Design review of the part built by this model. Coordinates are the model's own, in mm. A direction names the side the tool comes from. Round coordinates to 2 decimals unless told otherwise and drop trailing zeros. Write each loop counter-clockwise with the first axis right and the second up, starting at its lowest first coordinate (ties: lowest second). Pieces come first, ordered by that corner, then holes. Notation, with made-up numbers: (78.5, 51) - (98.5, 51) arc R17 cw to (98.5, 58) - close; hole circle Ø3 at (63, -26). An arc over 180 degrees is marked (long way). Use one line per item in the form item = value.
Autodesk Inventor part; units mm, degrees
ref_plane "h1_XY" through (-121.4374, 0, 0) normal (0, 1, 0) x (1, 0, 0)
ref_plane "h1_YZ" through (-121.4374, 0, 0) normal (1, 0, 0) x (0, 0, -1)
ref_plane "h1_ZX" through (-121.4374, 0, 0) normal (0, 0, -1) x (0, 1, 0)
sketch "Sketch_3" plane through (0, 0, 0) normal (0, 0, 1) x (1, 0, 0)
  line L0 (0, 0) -> (-121.4374, 0)
  line L1 (-121.4374, 0) -> (-121.4374, 1.9406)
  line L2 (-121.4374, 1.9406) -> (-120.965, 2.413)
  line L3 (-120.965, 2.413) -> (0, 2.413)
  line L4 (0, 2.413) -> (0, 0)
  line L5 (0, 0) -> (-121.4374, 0)
revolve "Revolution1" add sketch "Sketch_3" angle 360 about axis through (0, 0, 0) along (1, 0, 0)
thread "Thread1"
sketch "Sketch_17" plane through (0, 0, 0) normal (0, 0, 1) x (1, 0, 0)
  line L0 (121.4374, 0) -> (-121.4374, 0)
  line L1 (-108.9914, 2.413) -> (-108.9914, 2.159)
  line L2 (-108.9914, 2.159) -> (-108.7374, 2.159)
  line L3 (-108.7374, 2.159) -> (-108.7374, 2.413)
  line L4 (-108.7374, 2.413) -> (-108.9914, 2.413)
revolve "Revolution2" cut sketch "Sketch_17" angle 360 about axis through (121.4374, 0, 0) along (1, 0, 0)
sketch "Sketch_12" plane through (0, 0, 0) normal (0, 0, 1) x (1, 0, 0)
  line L0 (1.524, 0) -> (-15.875, 0)
  line L1 (-15.875, 0) -> (-15.875, 7.2771)
  line L2 (-15.875, 7.2771) -> (1.524, 7.2771)
  line L3 (1.524, 7.2771) -> (1.524, 0)
  line L4 (1.524, 0) -> (-15.875, 0)
revolve "Revolution3" add sketch "Sketch_12" angle 360 about axis through (1.524, 0, 0) along (1, 0, 0)
ref_plane "h1_XY" through (-121.4374, 0, 0) normal (0, 1, 0) x (1, 0, 0)
ref_plane "h1_YZ" through (-121.4374, 0, 0) normal (1, 0, 0) x (0, 0, -1)
ref_plane "h1_ZX" through (-121.4374, 0, 0) normal (0, 0, -1) x (0, 1, 0)
ref_plane "h2_XY" through (-108.7374, 0, 0) normal (0, 1, 0) x (1, 0, 0)
ref_plane "h2_YZ" through (-108.7374, 0, 0) normal (1, 0, 0) x (0, 0, -1)
ref_plane "h2_ZX" through (-108.7374, 0, 0) normal (0, 0, -1) x (0, 1, 0)
ref_plane "k1_XY" through (-121.4374, 0, -2.413) normal (0, 1, 0) x (1, 0, 0)
ref_plane "k1_YZ" through (-121.4374, 0, -2.413) normal (1, 0, 0) x (0, 0, -1)
ref_plane "k1_ZX" through (-121.4374, 0, -2.413) normal (0, 0, -1) x (0, 1, 0)
ref_plane "k2_XY" through (-121.4374, 0, 2.413) normal (0, 1, 0) x (1, 0, 0)
ref_plane "k2_YZ" through (-121.4374, 0, 2.413) normal (1, 0, 0) x (0, 0, -1)
ref_plane "k2_ZX" through (-121.4374, 0, 2.413) normal (0, 0, -1) x (0, 1, 0)
ref_plane "start_XY" through (-108.7374, 0, 0) normal (0, 1, 0) x (1, 0, 0)
ref_plane "start_YZ" through (-108.7374, 0, 0) normal (1, 0, 0) x (0, 0, -1)
ref_plane "start_ZX" through (-108.7374, 0, 0) normal (0, 0, -1) x (0, 1, 0)
ref_plane "to_prc_XY" through (-108.7374, 0, 0) normal (1, 0, 0) x (0, 0, -1)
ref_plane "to_prc_YZ" through (-108.7374, 0, 0) normal (0, 0, -1) x (0, 1, 0)
ref_plane "to_prc_ZX" through (-108.7374, 0, 0) normal (0, 1, 0) x (1, 0, 0)
ref_plane "to_rod_guide_XY" through (-121.4374, 0, 0) normal (1, 0, 0) x (0, 0, -1)
ref_plane "to_rod_guide_YZ" through (-121.4374, 0, 0) normal (0, 0, -1) x (0, 1, 0)
ref_plane "to_rod_guide_ZX" through (-121.4374, 0, 0) normal (0, 1, 0) x (1, 0, 0)
properties part number "D-75080.5-2XP-4.781-3pos"
Q1. Machinability: for faces 1 (the cylindrical face through (-7.05, 6.94, 2.19)), 2 (the cylindrical face through (-61.656, -1.915, -1.468)), which of the approach directions +Z, -Z, +X, -X, +Y, -Y give a long, thin tool a straight path to every point of the face, cutting with its end or side? Answer none if there is none.
Calculated:
face_1 = +X, -X
face_2 = -X
Q2. We need section A-A on y = 0. Write out the cut boundary in (x, z) (3 decimals).
Calculated:
outline = (-121.437, -1.941) - (-120.965, -2.413) - (-108.991, -2.413) - (-108.991, -2.159) - (-108.737, -2.159) - (-108.737, -2.413) - (-15.875, -2.413) - (-15.875, -7.277) - (1.524, -7.277) - (1.524, 7.277) - (-15.875, 7.277) - (-15.875, 2.413) - (-108.737, 2.413) - (-108.737, 2.159) - (-108.991, 2.159) - (-108.991, 2.413) - (-120.965, 2.413) - (-121.437, 1.941) - close
Q3. For P1, Ø5, axis at x = -55.5, z = 1.5, coming from the +Y side; P2, Ø3, axis at x = -101, z = -2.5, coming from the +Y side, all flat-tipped, find the tip position at first contact; note any pin that passes through.
Calculated:
P1 = 2.41
P2 = 2.2
Q4. We need section D-D on y = 5.5. Write out the cut boundary in (x, z) (3 decimals).
Calculated:
outline = (-15.875, -4.765) - (1.524, -4.765) - (1.524, 4.765) - (-15.875, 4.765) - close
Q5. We need section C-C on x = -51. Write out the cut boundary in (y, z), then the cut area to 3 significant figures.
Calculated:
outline = circle Ø4.83 at (0, 0)
area = 18.3 mm2
Q6. To check wall thickness, follow line 1 along X through (y, z) = (0.5, -5.75) (3 decimals); line 2 along Z through (x, y) = (-80.5, 0.25). State the ranges of each line that lie inside material, in increasing order. Write a range as from..to.
Calculated:
line_1 = -15.875..1.524
line_2 = -2.4..2.4
